Autodesk Inventor part; units mm, degrees
ref_plane "YZ Plane" through (0, 0, 0) normal (1, 0, 0) x (0, 1, 0)
ref_plane "XZ Plane" through (0, 0, 0) normal (0, 1, 0) x (-1, 0, 0)
ref_plane "XY Plane" through (0, 0, 0) normal (0, 0, 1) x (1, 0, 0)
sketch "Sketch1" plane through (0, 0, 0) normal (0, 1, 0) x (-1, 0, 0)
  circle A0 centre (0, 0) radius 1.125
  circle A1 centre (0, 0) radius 2.5
  dimension "d0" = 2.25
  dimension "d1" = 5
extrude "Extrusion1" add sketch "Sketch1" along normal blind 9
sketch "Sketch2" plane through (0, 0, 0) normal (0, 0, 1) x (1, 0, 0)
  line L0 (2.5, 9) -> (-2.5, 9)
  line L1 (2.5, 0) -> (-2.5, 0)
  line L2 (-2.5, 0) -> (-2.5, 9)
  line L3 (-2.5, 7) -> (2.5173, 7)
  line L4 (2.5, 9) -> (-2.5, 9)
  line L5 (0, 9) -> (0, 0)
  circle A0 centre (0, 4.9) radius 2.1
  dimension "d4" = 2
  dimension "d5" = 4.2
extrude "Extrusion2" cut sketch "Sketch2" along normal blind 12 contours A0 L5 | L5 A0
sketch "Sketch3" plane through (0, 0, 0) normal (1, 0, 0) x (0, 1, 0)
  line L0 (9, -2.5) -> (9, 2.5)
  line L1 (0, -2.5) -> (0, 2.5)
  line L2 (0, 2.5) -> (9, 2.5)
  line L3 (7, 2.5) -> (7, -2.525)
  line L4 (9, 1.125) -> (9, -1.125)
  line L5 (9, 0) -> (0, 0)
  circle A0 centre (4.9, 0) radius 2.1
  point P0 (4.9, 1.3565)
  dimension "d8" = 2
  dimension "d9" = 4.2
extrude "Extrusion3" cut sketch "Sketch3" along normal up to next contours A0 L5 | L5 A0
properties part number "motor_shaft_adapter" material "ABS Plastic"
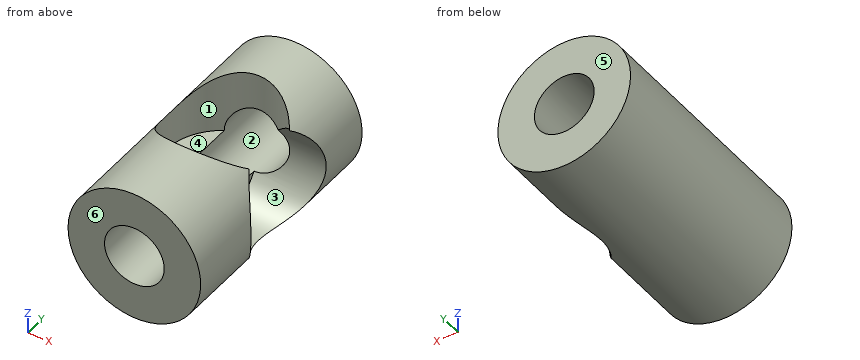
The listing builds one solid part. Answer for the finished solid, in the listing's coordinates (mm). Face numbers are marked on the shaded views. A direction names the side the tool comes from. Round coordinates to 2 decimals unless told otherwise and drop trailing zeros. Write each loop counter-clockwise with the first axis right and the second up, starting at its lowest first coordinate (ties: lowest second). Pieces come first, ordered by that corner, then holes. Notation, with made-up numbers: (23.25, -17) - (51.25, -17) arc R8 cw to (51.25, -9) - close; hole circle Ø5 at (55, -19.75). An arc over 180 degrees is marked (long way). Use a Markdown table: item, result. Add a question column.
1. Consider line 1 (Z direction, x = 0.05, y = 1.5); line 2 (Z direction, x = -0.5, y = 2); line 3 (Y direction, x = 0.8, z = 1.15). Determine where each line is inside the solid, lowest interval first.
2. A flat-ended cylindrical pin translates along its axis: P1, Ø0.5, axis at y = 4, z = -1.5, coming from the +X side. Find the tip coordinate at first contact, or state that the pin passes through.
3. The part is cut by section D-D (y = 5.75). Write down the section's boundary in (x, z) (3 decimals), and give its area (3 significant figures).
4. The part is cut by section C-C (x = 1.6). Write down the section's boundary in (y, z), and give its area (3 significant figures).
5. A tool of negligible diameter and unlimited length cuts with its end or side. For the marked faces 1 and 2, from which of +Z, -Z, +X, -X, +Y, -Y can it reach the whole face along a straight path? Write none if from no direction.
6. The part is cut by section A-A (x = 0.9). Write down the section's boundary in (y, z) (3 decimals), and give its area (3 significant figures).
7. The part is cut by section B-B (y = 8.75). Write down the section's boundary in (x, z) (3 decimals), and give its area (3 significant figures).
8. For a pull along Y with two mould halves and no side action, classify the marked faces 3, 4, 5 and 6 as +Y half, -Y half, draft (parallel to the pull), parting line (faces both ways), or undercut.
Reported:
| question | item | result |
|---|---|---|
| 1 | line 1 | -2.5 to -1.12, 1.12 to 2.5 |
| 1 | line 2 | -2.45 to -1.01, 1.01 to 2.45 |
| 1 | line 3 | 0 to 2.96, 6.84 to 9 |
| 2 | P1 | x = 0 |
| 3 | outline | (-1.92, 0) - (-1.92, 1.601) arc R2.5 ccw to (1.601, -1.92) - (0, -1.92) - (0, -1.125) arc R1.125 cw to (-1.125, 0) - close |
| 3 | area | 5.18 mm^2 |
| 4 | outline | (0, -1.92) - (4.05, -1.92) arc R2.1 cw to (3.54, 1.6) - (3.54, 1.92) - (0, 1.92) - close; (5.75, -1.92) - (9, -1.92) - (9, 1.92) - (6.26, 1.92) - (6.26, 1.6) arc R2.1 cw to start |
| 4 | area | 21.0 mm^2 |
| 5 | face 1 | +Z |
| 5 | face 2 | +Y, -Y |
| 6 | outline | (0, -2.332) - (9, -2.332) - (9, -0.675) - (6.889, -0.675) arc R2.1 cw to (2.911, -0.675) - (0, -0.675) - close; (0, 0.675) - (2.911, 0.675) arc R2.1 cw to (3.003, 0.9) - (3.003, 2.332) - (0, 2.332) - close; (6.797, 0.9) arc R2.1 cw to (6.889, 0.675) - (9, 0.675) - (9, 2.332) - (6.797, 2.332) - close |
| 6 | area | 19.4 mm^2 |
| 7 | outline | circle Ø5 at (0, 0); hole circle Ø2.25 at (0, 0) |
| 7 | area | 15.7 mm^2 |
| 8 | face 3 | undercut |
| 8 | face 4 | undercut |
| 8 | face 5 | +Y half |
| 8 | face 6 | -Y half |
